Source: CAD feature listing. Evaluate the final solid. Frame: model axes, mm. A direction names the side the tool comes from. Coordinates: 2 decimals unless noted, no trailing zeros. Order: outer loops, then holes, each group sorted by start corner. A loop starts at its lowest first (then second) coordinate and runs counter-clockwise, first axis right, second up.
Item 1: Section C-C on y = -4.25. Return the cut outline in (x, z), then the cut area to 3 significant figures.
Item 2: Section A-A on z = 27. Return the cut outline in (x, y), then the cut area to 3 significant figures.
Item 3: Ray query, line 1 (Y direction, x = -0.25, z = 75.5); line 2 (Y direction, x = -5.5, z = 25); line 3 (X direction, y = 1.75, z = 93). Return the intervals inside material, ascending.
Item 4: Reachability of faces 1 (the flat face through (-3, -6, 100.012)), 2 (the flat face through (3, 6, 100.012)), 3 (the cylindrical face through (4.29, 4.68, 103.93)), 4 (the flat face through (7, 0, 100.012)) from +Z, -Z, +X, -X, +Y, -Y: full face, straight path, thin tool, end or side. Return the list, or none.
Item 5: Mould query, pull axis Y, two halves, no side actions, for faces 5 (the flat face through (-5.525, -3.131, 49.306)), 6 (the cylindrical face through (0.336, -2.558, 53.219)), 7 (the flat face through (-3, 6, 100.012)). Classes: released by +Y, released by -Y, zero draft, split by the parting line, or undercut.
Item 6: Section B-B on x = -1.25. Return the cut outline in (y, z).
Item 7: Contact query for a flat-ended pin moving along its axis: P1, Ø3, axis at y = -3, z = 59.5, coming from the +X side. Output: stop coordinate, or through.
from build123d import *

# Parameters (mm, degrees)
SKETCH1_R           = 2.5796875
BOSS_EXTRUDE1_DEPTH = 100.0125
SKETCH2_R           = 6.35
SKETCH2_R_2         = 2.5796875
BOSS_EXTRUDE2_DEPTH = 7.9375


with BuildPart() as part:
    # Sketch1 → Boss-Extrude1 (new body)
    with BuildSketch(Plane.XY):
        Polygon((7.332348419, 0), (3.666174209, 6.35), (-3.666174209, 6.35), (-7.332348419, 0), (-3.666174209, -6.35), (3.666174209, -6.35), align=None)
        with Locations(Location((0, 0, 0), (0, 0, 180))):
            Circle(SKETCH1_R, mode=Mode.SUBTRACT)
    extrude(amount=BOSS_EXTRUDE1_DEPTH)

    # Sketch2 → Boss-Extrude2 (add)
    with BuildSketch(Plane.XY.offset(100.0125)):
        with Locations(Location((0, 0, 0), (0, 0, 150))):
            Circle(SKETCH2_R)
        with Locations(Location((0, 0, 0), (0, 0, 180))):
            Circle(SKETCH2_R_2, mode=Mode.SUBTRACT)
    extrude(amount=BOSS_EXTRUDE2_DEPTH)


solid = part.part
Answer list:
1. outline: (-4.88, 0) - (4.88, 0) - (4.88, 100.01) - (4.72, 100.01) - (4.72, 107.95) - (-4.72, 107.95) - (-4.72, 100.01) - (-4.88, 100.01) - close
1. area: 1,050 mm2
2. outline: (-7.33, 0) - (-3.67, -6.35) - (3.67, -6.35) - (7.33, 0) - (3.67, 6.35) - (-3.67, 6.35) - close; hole circle Ø5.16 at (0, 0)
2. area: 119 mm2
3. line 1: y = -6.35 to -2.57, 2.57 to 6.35
3. line 2: y = -3.17 to 3.17
3. line 3: x = -6.32 to -1.9, 1.9 to 6.32
4. face 1: +Z, -X, -Y
4. face 2: +Z, +X, +Y
4. face 3: +Z
4. face 4: +Z, +X
5. face 5: released by -Y
5. face 6: undercut
5. face 7: zero draft
6. outline: (-6.35, 0) - (-2.26, 0) - (-2.26, 107.95) - (-6.23, 107.95) - (-6.23, 100.01) - (-6.35, 100.01) - close; (2.26, 0) - (6.35, 0) - (6.35, 100.01) - (6.23, 100.01) - (6.23, 107.95) - (2.26, 107.95) - close
7. P1: stops at x = 6.47
